Work out the finished part from the listing and answer in its coordinate system (mm). A direction names the side the tool comes from. Round coordinates to 2 decimals unless told otherwise and drop trailing zeros. Loops run counter-clockwise (first coordinate to the right, second up) from the corner with the lowest first, then second, coordinate; pieces in that order, holes last. Notation, with made-up numbers: (75.25, 69.25) - (120.25, 69.25) arc R18 cw to (120.25, 98.25) - close; hole circle Ø11 at (47, -33.5). An arc over 180 degrees is marked (long way). Return JSON: item names as keys, results as strings.
from build123d import *

# Parameters (mm, degrees)
SKETCH1_W              = 8.5
SKETCH1_H              = 12
BOSS_EXTRUDE1_DEPTH    = 41.5
CUT_EXTRUDE1_DEPTH     = 43.784342931
FILLET1_R              = 0.5
M2_HOLE1_J_D           = 2.4
M2_HOLE1_J_DEPTH       = 5
M2_HOLE1_J_TIP         = 0.721032743
M2_HOLE2_K_D           = 2.4
M2_HOLE2_K_CSINK_D     = 4.4
M2_HOLE2_K_CSINK_ANGLE = 90
M2_HOLE3_L_D           = 2.4
M2_HOLE3_L_DEPTH       = 10
M2_HOLE3_L_TIP         = 0.721032743
M2_HOLE4_M_D           = 2.4
M2_HOLE5_N_D           = 2.4
M2_HOLE5_N_DEPTH       = 4
M2_HOLE5_N_TIP         = 0.721032743
M2_HOLE6_P_D           = 2.4
M2_HOLE6_P_DEPTH       = 10
M2_HOLE6_P_TIP         = 0.721032743


with BuildPart() as part:
    # Sketch1 → Boss-Extrude1 (new, symmetric)
    with BuildSketch(Plane.XY):
        Rectangle(SKETCH1_W, SKETCH1_H)
    extrude(amount=BOSS_EXTRUDE1_DEPTH, both=True)

    # Sketch2 → Cut-Extrude1 (cut, through all)
    with BuildSketch(Plane(origin=(4.25, 0, 0), x_dir=(0, 0, -1), z_dir=(1, 0, 0))):
        with BuildLine():
            Line((-37.5, 1), (37.5, 1))
            ThreePointArc((37.5, 1), (38.207106781, 0.707106781), (38.5, 0))
            Line((38.5, 0), (38.5, -6))
            Line((38.5, -6), (-38.5, -6))
            Line((-38.5, -6), (-38.5, 0))
            ThreePointArc((-38.5, 0), (-38.207106781, 0.707106781), (-37.5, 1))
        make_face()
    extrude(amount=-CUT_EXTRUDE1_DEPTH, mode=Mode.SUBTRACT)

    # Fillet1
    fillet1_edges = [part.edges().sort_by_distance(p)[0] for p in [
        (0, -6, 41.5),
        (0, -6, -38.5),
        (0, -6, 38.5),
        (0, -6, -41.5),
        (0, 6, -41.5),
        (0, 6, 41.5),
    ]]
    fillet(fillet1_edges, radius=FILLET1_R)

    # M2 Hole1 - J
    with Locations(Plane(origin=(4.25, 0, 0), x_dir=(0, 0, -1), z_dir=(1, 0, 0))):
        with Locations((-35.5, 3.5), (35.5, 3.5)):
            Hole(M2_HOLE1_J_D / 2, depth=M2_HOLE1_J_DEPTH)
            with Locations((0, 0, -(M2_HOLE1_J_DEPTH + M2_HOLE1_J_TIP / 2))):  # 118° drill point
                Cone(0, M2_HOLE1_J_D / 2, M2_HOLE1_J_TIP, mode=Mode.SUBTRACT)

    # M2 Hole2 - K (through all)
    with Locations(Plane(origin=(4.25, 0, 0), x_dir=(0, 0, -1), z_dir=(1, 0, 0))):
        with Locations((-21.5, 3.5), (21.5, 3.5)):
            CounterSinkHole(M2_HOLE2_K_D / 2, M2_HOLE2_K_CSINK_D / 2, counter_sink_angle=M2_HOLE2_K_CSINK_ANGLE)

    # M2 Hole3 - L
    with Locations(Plane.XY.offset(41.5)):
        with Locations((0, -3)):
            Hole(M2_HOLE3_L_D / 2, depth=M2_HOLE3_L_DEPTH)
            with Locations((0, 0, -(M2_HOLE3_L_DEPTH + M2_HOLE3_L_TIP / 2))):  # 118° drill point
                Cone(0, M2_HOLE3_L_D / 2, M2_HOLE3_L_TIP, mode=Mode.SUBTRACT)

    # M2 Hole4 - M (through all)
    with Locations(Plane(origin=(0, 6, 0), x_dir=(1, 0, 0), z_dir=(0, 1, 0))):
        with Locations((0, 29), (0, -29)):
            Hole(M2_HOLE4_M_D / 2)

    # M2 Hole5 - N
    with Locations(Plane.ZY.offset(4.25)):
        with Locations((0, 3.5)):
            Hole(M2_HOLE5_N_D / 2, depth=M2_HOLE5_N_DEPTH)
            with Locations((0, 0, -(M2_HOLE5_N_DEPTH + M2_HOLE5_N_TIP / 2))):  # 118° drill point
                Cone(0, M2_HOLE5_N_D / 2, M2_HOLE5_N_TIP, mode=Mode.SUBTRACT)

    # M2 Hole6 - P
    with Locations(Plane(origin=(0, 0, -41.5), x_dir=(-1, 0, 0), z_dir=(0, 0, -1))):
        with Locations((0, -3)):
            Hole(M2_HOLE6_P_D / 2, depth=M2_HOLE6_P_DEPTH)
            with Locations((0, 0, -(M2_HOLE6_P_DEPTH + M2_HOLE6_P_TIP / 2))):  # 118° drill point
                Cone(0, M2_HOLE6_P_D / 2, M2_HOLE6_P_TIP, mode=Mode.SUBTRACT)


solid = part.part
1) Section A-A (x = -3) is taken. Give the vertices of the cut face in (y, z).
Verdict:
{"outline": "(-6, -41) arc R0.5 ccw to (-5.5, -41.5) - (5.5, -41.5) arc R0.5 ccw to (6, -41) - (6, 41) arc R0.5 ccw to (5.5, 41.5) - (-5.5, 41.5) arc R0.5 ccw to (-6, 41) - (-6, 39) arc R0.5 ccw to (-5.5, 38.5) - (0, 38.5) arc R1 cw to (1, 37.5) - (1, -37.5) arc R1 cw to (0, -38.5) - (-5.5, -38.5) arc R0.5 ccw to (-6, -39) - close; hole circle Ø2.4 at (3.5, -21.5); hole circle Ø2.4 at (3.5, 0); hole circle Ø2.4 at (3.5, 21.5)"}
2) Find the intervals of material crossed by L1, parallel to Z at x = -2, y = 3.5; L2, parallel to Z at x = 0, y = -4.25; L3, parallel to Y at x = 1.75, z = -21.5, in increasing order.
Verdict:
{"L1": "z = -41.5 to -22.7, -20.3 to -1.2, 1.2 to 20.3, 22.7 to 41.5", "L2": "z = -41.5 to -38.5, 38.5 to 41.5", "L3": "y = 1 to 2.3, 4.7 to 6"}
3) Section B-B (y = -3) is taken. Give the vertices of the cut face in (x, z).
Verdict:
{"outline": "(-4.25, -41.5) - (-1.2, -41.5) - (-1.2, -38.5) - (-4.25, -38.5) - close; (-4.25, 38.5) - (-1.2, 38.5) - (-1.2, 41.5) - (-4.25, 41.5) - close; (1.2, -41.5) - (4.25, -41.5) - (4.25, -38.5) - (1.2, -38.5) - close; (1.2, 38.5) - (4.25, 38.5) - (4.25, 41.5) - (1.2, 41.5) - close"}
4) Section D-D (z = 17) is taken. Give the vertices of the cut face in (x, y).
Verdict:
{"outline": "(-4.25, 1) - (4.25, 1) - (4.25, 6) - (-4.25, 6) - close"}
5) Section C-C (z = -21.5) is taken. Give the vertices of the cut face in (x, y), and give its area (3 significant figures).
Verdict:
{"outline": "(-4.25, 1) - (4.25, 1) - (4.25, 1.3) - (3.25, 2.3) - (-4.25, 2.3) - close; (-4.25, 4.7) - (3.25, 4.7) - (4.25, 5.7) - (4.25, 6) - (-4.25, 6) - close", "area": "21.1 mm2"}
6) Flat-ended cylindrical pins translate along their axes: pin 1 (5 mm diameter, centred on x = -0.5, z = 14, fed in from -Y); pin 2 (3 mm diameter, centred on y = 3.5, z = -21.5, fed in from +X); pin 3 (1.4 mm diameter, centred on x = 0, y = -3, fed in from +Z). Find the tip coordinate at first contact, or state that the pin passes through.
Verdict:
{"pin 1": "stops at y = 1", "pin 2": "stops at x = 3.55", "pin 3": "passes through"}
7) A tool of negligible diameter and unlimited length cuts with its end or side. For faces 1 (the cylindrical face through (-2.22, 2.33, 0.26)), 2 (the flat face through (0, 6, 1)), 3 (the cylindrical face through (1.72, 3.04, 36.61)), 4 (the flat face through (1, -2, -38.5)), from which of +Z, -Z, +X, -X, +Y, -Y can it reach the whole face along a straight path? Write none if from no direction.
Verdict:
{"face 1": "-X", "face 2": "+Z, -Z, +X, -X, +Y", "face 3": "+X", "face 4": "+X, -X, -Y"}
8) Determine the mould class of faces 5 (the flat face through (0, 0, 41.5)), 6 (the cylindrical face through (-0.554, 3.465, 30.065)), 7 (the conical face through (-1.346, 3.509, -35.292)) for opening direction X: pulls with the +X half, pulls with the -X half, needs draft (parallel to the pull), parting line crosses it, or undercut.
Verdict:
{"face 5": "needs draft", "face 6": "undercut", "face 7": "pulls with the +X half"}
